Read the model definition and answer for the solid it produces. Units are mm, in the model's axes. A direction names the side the tool comes from. Round coordinates to 2 decimals unless told otherwise and drop trailing zeros. Order: outer loops, then holes, each group sorted by start corner. A loop starts at its lowest first (then second) coordinate and runs counter-clockwise, first axis right, second up.
from build123d import *

# Parameters (mm, degrees)
F0_W     = 50
F0_H     = 50
F1_DEPTH = 50
F3_DEPTH = 40
F4_R     = 3.139309
F5_DEPTH = 25


with BuildPart() as f1:
    # F0 (on Top) → F1 (new body)
    with BuildSketch(Plane.XY):
        with Locations((1.594128, -1.850611)):
            Rectangle(F0_W, F0_H)
    extrude(amount=F1_DEPTH)

    # F2 (on face) → F3 (cut)
    with BuildSketch(Plane.XY.offset(50)):
        Polygon((-5.974522, -15.155445), (11.525478, -15.155445), (20.275478, 0), (11.525478, 15.155445), (-5.974522, 15.155445), (-14.724522, 0), align=None)
    extrude(amount=-F3_DEPTH, mode=Mode.SUBTRACT)

    # F4 (on face) → F5 (join)
    with BuildSketch(Plane.XY.offset(10)):
        with Locations((3.275001, 2.058548)):
            Circle(F4_R)
    extrude(amount=F5_DEPTH)


solid = f1.part
Q1. For faces 1 (the face through (-10.29, 7.68, 30.28)), 2 (the face through (26.594, -2, 25)), determine the directions among +Z, -Z, +X, -X, +Y, -Y from which every point of the face is accessible in a straight line to the end or side of a thin tool.
Outcome:
face 1: +Z
face 2: +Z, -Z, +X, +Y, -Y
Q2. A cutting plane is placed at B-B, the plane x = -3.5. Give the vertices of the cut face in (y, z), plus the area to 3 significant figures.
Outcome:
outline: (-26.85, 0) - (23.15, 0) - (23.15, 50) - (15.16, 50) - (15.16, 10) - (-15.16, 10) - (-15.16, 50) - (-26.85, 50) - close
area: 1,290 mm2
Q3. A cutting plane is placed at A-A, the plane z = 32. Give the vertices of the cut face in (x, y) (3 decimals).
Outcome:
outline: (-23.406, -26.851) - (26.594, -26.851) - (26.594, 23.149) - (-23.406, 23.149) - close; circle Ø6.279 at (3.275, 2.059); hole (-14.725, 0) - (-5.975, -15.155) - (11.525, -15.155) - (20.275, 0) - (11.525, 15.155) - (-5.975, 15.155) - close
Q4. A cutting plane is placed at C-C, the plane z = 37.5. Give the vertices of the cut face in (x, y), plus the area to 3 significant figures.
Outcome:
outline: (-23.41, -26.85) - (26.59, -26.85) - (26.59, 23.15) - (-23.41, 23.15) - close; hole (-14.72, 0) - (-5.97, -15.16) - (11.53, -15.16) - (20.28, 0) - (11.53, 15.16) - (-5.97, 15.16) - close
area: 1,700 mm2
Q5. Straight lines are drawn through the part: probe 1 along Y at (x, z) = (8.5, 16); probe 2 along Y at (x, z) = (0.5, 25); probe 3 along Z at (x, y) = (-6.5, 7.5). For each, find the intervals that lie inside material, in ascending order.
Outcome:
probe 1: y = -26.85 to -15.16, 15.16 to 23.15
probe 2: y = -26.85 to -15.16, 0.59 to 3.53, 15.16 to 23.15
probe 3: z = 0 to 10
Q6. For a pull along Y with two mould halves and no side action, classify faces 3 (the face through (3, 2, 35)), 4 (the face through (1, -26.851, 25)), 5 (the face through (-10, -13, 50)) as released by +Y, released by -Y, zero draft, split by the parting line, or undercut.
Outcome:
face 3: undercut
face 4: released by -Y
face 5: zero draft
Q7. A cutting plane is placed at D-D, the plane y = 3. Give the vertices of the cut face in (x, z).
Outcome:
outline: (-23.41, 0) - (26.59, 0) - (26.59, 50) - (18.54, 50) - (18.54, 10) - (6.27, 10) - (6.27, 35) - (0.28, 35) - (0.28, 10) - (-12.99, 10) - (-12.99, 50) - (-23.41, 50) - close
Q8. A flat-ended cylindrical pin translates along its axis: pin 1 (15 mm diameter, centred on x = -4.5, y = 1, fed in from +Z). Find the tip coordinate at first contact, or state that the pin passes through.
Outcome:
pin 1: stops at z = 35
